Here's the drawing with two shaded views (mm, measured from the low corner). I have some questions. A direction names the side the tool comes from. Give positions to 0.01 mm unless a question says otherwise; leave off trailing zeros. Loops run counter-clockwise (first coordinate to the right, second up) from the corner with the lowest first, then second, coordinate; pieces in that order, holes last. Notation, with made-up numbers: M -11.75,81 L 36.25,81 A12 cw 36.25,92 Z; hole C -34.75,-11 d4. An arc over 180 degrees is marked long. Put each result on its own line as item: value. Start each with the question number.
1) Imagine slicing it at A-A (x = 4). Write out the boundary of the cut face in (y, z).
2) Imagine slicing it at C-C (y = 3). Write out the boundary of the cut face in (x, z), then the cut area to 3 significant figures.
3) For P1, Ø6, axis at y = 26, z = 18, coming from the +X side; P2, Ø6, axis at x = 27, z = 24, coming from the +Y side, each with a flat end and sliding along its axis, tell me the tip position at first contact or that it passes through.
4) Please list where these lines run through material, in increasing order: line 1 along Y through (x, z) = (16, 2.5); line 2 along X through (y, z) = (6, 6); line 3 along X through (y, z) = (6.5, 7). Write a range as from..to.
5) If we mould it in two halves opening along X, with no side actions, what happens to the marked faces 1, 2 and 3? For each: +X half, -X half, draft (parallel to the pull), parting line (faces both ways), or undercut.
6) For the marked faces 4 and 5, which set-ups out of +Z, -Z, +X, -X, +Y, -Y let a thin tool reach every point of the face, with its end or its side?
7) Imagine slicing it at B-B (z = 8). Write out the boundary of the cut face in (x, y) (3 decimals), then the cut area to 3 significant figures.
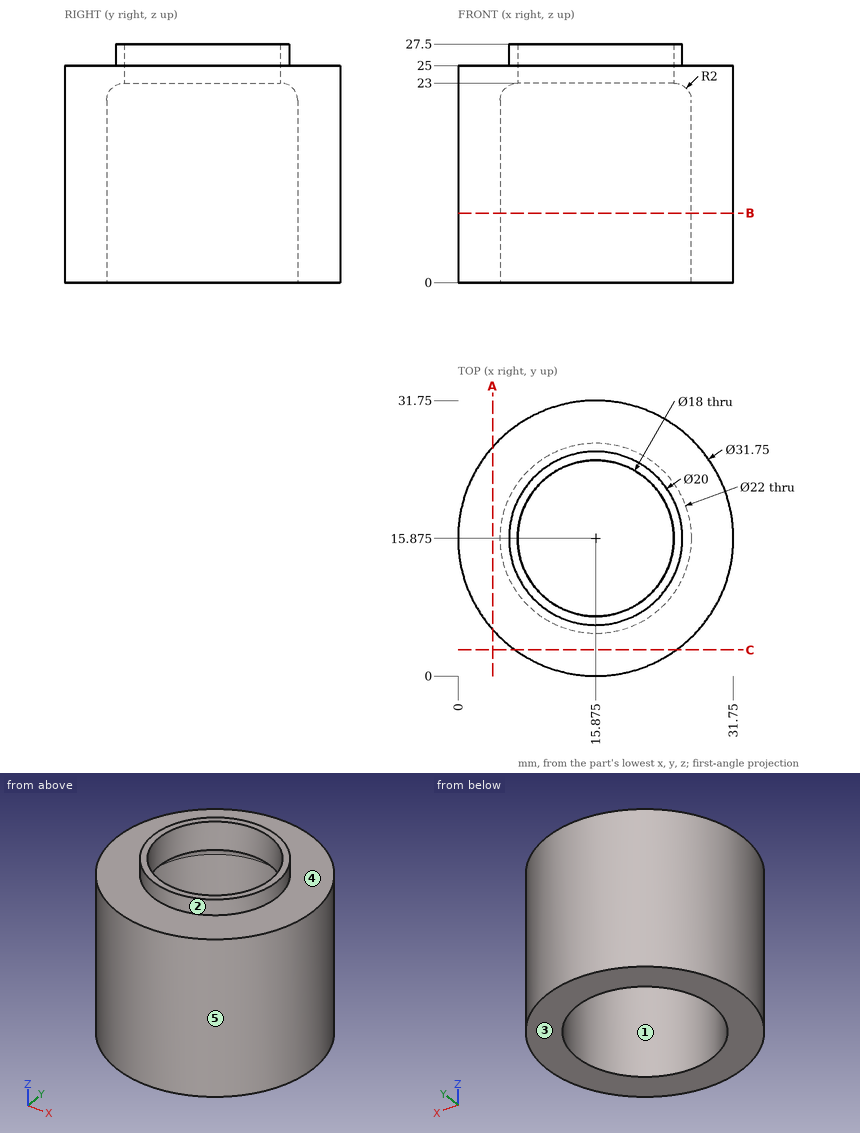
Recorded:
1. outline: M 5.34,0 L 26.41,0 L 26.41,25 L 5.34,25 Z
2. outline: M 6.59,0 L 25.16,0 L 25.16,25 L 6.59,25 Z
2. area: 464 mm²
3. P1: x = 30.06
3. P2: y = 29.51
4. line 1: 0..4.88, 26.87..31.75
4. line 2: 3.45..11.03, 20.72..28.3
4. line 3: 3.06..10.12, 21.63..28.69
5. face 1: undercut
5. face 2: parting line
5. face 3: draft
6. face 4: +Z
6. face 5: +Z, -Z
7. outline: C 15.875,15.875 d31.75; hole C 15.875,15.875 d22
7. area: 412 mm²
